Verification items for this drawing (mm, ordinates from the low corner). Round coordinates to 2 decimals unless told otherwise and drop trailing zeros. Loops run counter-clockwise (first coordinate to the right, second up) from the corner with the lowest first, then second, coordinate; pieces in that order, holes last. Notation, with made-up numbers: (-34, 55) -> (15, 55) arc R26 cw to (15, 72) -> close; hole circle Ø5 at (53, 33). An arc over 180 degrees is marked (long way). One line per question, with ' | ' between items.
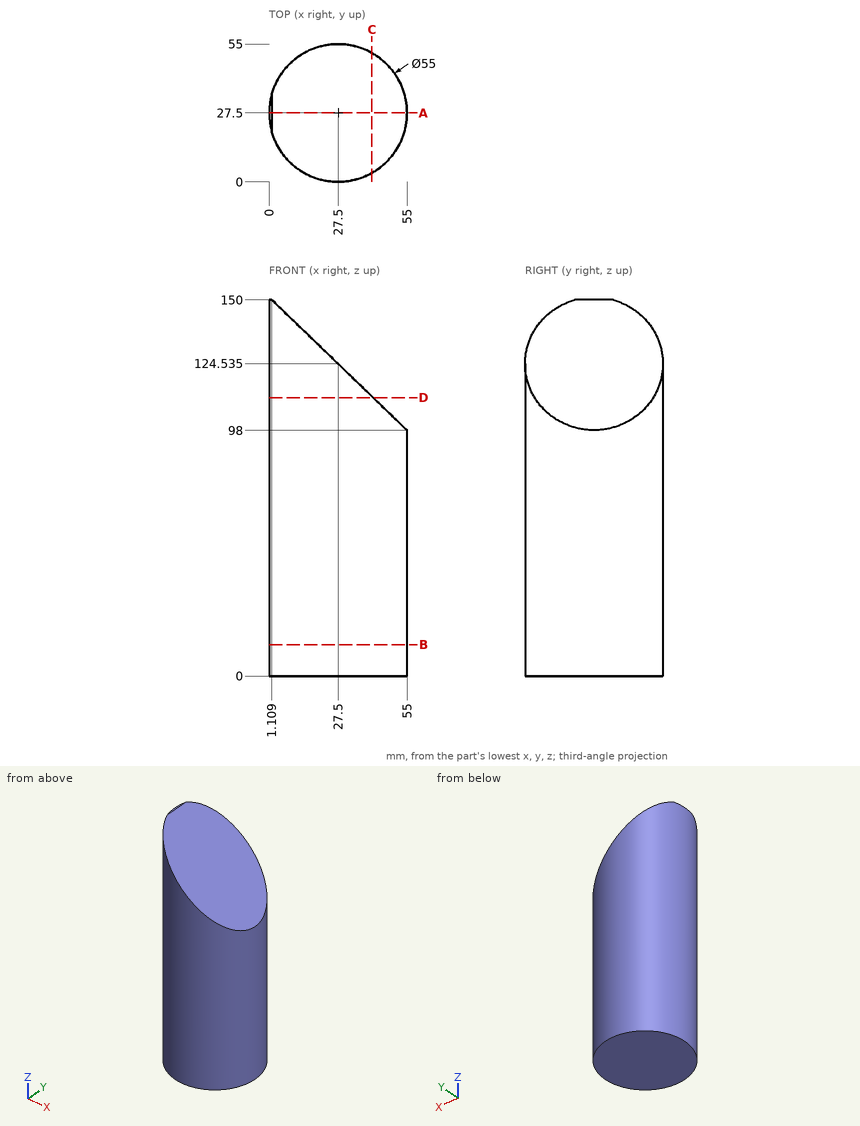
(1) Scan lines: probe 1 along X at (y, z) = (28, 73.5); probe 2 along X at (y, z) = (21, 33); probe 3 along Y at (x, z) = (24.5, 75). Record each from-to range of solid material in increasing order.
Answer:
probe 1: x = 0 to 55 | probe 2: x = 0.78 to 54.22 | probe 3: y = 0.16 to 54.84
(2) Sectioned sample at A-A, the plane y = 27.5. Record the cut outline in (x, z).
Answer:
outline: (0, 0) -> (55, 0) -> (55, 98) -> (1.11, 150) -> (0, 150) -> close
(3) Go/stop test with flat-tipped pins: pin 1 (5 mm diameter, centred on x = 36, z = 113, fed in from -Y); pin 2 (4 mm diameter, centred on x = 36, y = 44, fed in from +Z); pin 3 (1.5 mm diameter, centred on y = 25, z = 28.5, fed in from -X). Record where each tip stops, or that it passes through.
Answer:
pin 1: stops at y = 0.66 | pin 2: stops at z = 118.26 | pin 3: stops at x = 0.06
(4) Sectioned sample at D-D, the plane z = 111. Record the cut outline in (x, y), and give its area (3 significant figures).
Answer:
outline: (41.53, 3.85) -> (41.53, 51.15) arc R27.5 ccw (long way) to start | area: 1,920 mm2
(5) Sectioned sample at B-B, the plane z = 12.5. Record the cut outline in (x, y).
Answer:
outline: circle Ø55 at (27.5, 27.5)
(6) Sectioned sample at C-C, the plane x = 41. Record the cut outline in (y, z), and give its area (3 significant figures).
Answer:
outline: (3.54, 0) -> (51.46, 0) -> (51.46, 111.51) -> (3.54, 111.51) -> close | area: 5,340 mm2
